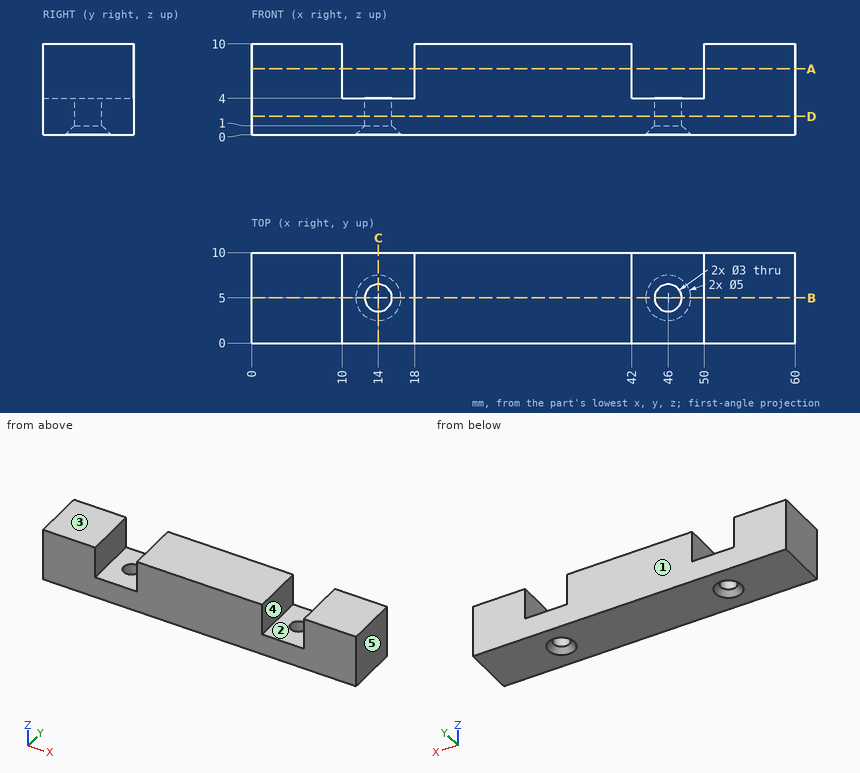
Here's the drawing with two shaded views (mm, measured from the low corner). I have some questions. A direction names the side the tool comes from. Coordinates: 2 decimals unless noted, no trailing zeros. Order: outer loops, then holes, each group sorted by start corner. A loop starts at its lowest first (then second) coordinate and runs counter-clockwise, first axis right, second up.
Item 1: For the marked faces 1 and 2, which set-ups out of +Z, -Z, +X, -X, +Y, -Y let a thin tool reach every point of the face, with its end or its side?
Result sheet:
face 1: +Z, -Z, +X, -X, +Y
face 2: +Z, +Y, -Y
Item 2: For P1, Ø4, axis at x = 13.5, y = 4.5, coming from the +Z side; P2, Ø3, axis at y = 7.5, z = 8, coming from the -X side, each with a flat end and sliding along its axis, tell me the tip position at first contact or that it passes through.
Result sheet:
P1: stops at z = 4
P2: stops at x = 0
Item 3: If we section it at D-D on z = 2: List the corners of the cut face in (x, y) for me.
Result sheet:
outline: (0, 0) - (60, 0) - (60, 10) - (0, 10) - close; hole circle Ø3 at (14, 5); hole circle Ø3 at (46, 5)
Item 4: If we section it at C-C on x = 14: List the corners of the cut face in (y, z) for me, plus the area to 3 significant figures.
Result sheet:
outline: (0, 0) - (2.5, 0) - (3.5, 1) - (3.5, 4) - (0, 4) - close; (6.5, 1) - (7.5, 0) - (10, 0) - (10, 4) - (6.5, 4) - close
area: 27.0 mm2
Item 5: If we section it at B-B on y = 5: List the corners of the cut face in (x, z) for me, plus the area to 3 significant figures.
Result sheet:
outline: (0, 0) - (11.5, 0) - (12.5, 1) - (12.5, 4) - (10, 4) - (10, 10) - (0, 10) - close; (15.5, 1) - (16.5, 0) - (43.5, 0) - (44.5, 1) - (44.5, 4) - (42, 4) - (42, 10) - (18, 10) - (18, 4) - (15.5, 4) - close; (47.5, 1) - (48.5, 0) - (60, 0) - (60, 10) - (50, 10) - (50, 4) - (47.5, 4) - close
area: 478 mm2
Item 6: If we section it at A-A on z = 7.25: List the corners of the cut face in (x, y) for me, plus the area to 3 significant figures.
Result sheet:
outline: (0, 0) - (10, 0) - (10, 10) - (0, 10) - close; (18, 0) - (42, 0) - (42, 10) - (18, 10) - close; (50, 0) - (60, 0) - (60, 10) - (50, 10) - close
area: 440 mm2
Item 7: I need wall thicknesses on line 1 (X direction, y = 3, z = 8); line 2 (X direction, y = 5, z = 2.15); line 3 (Y direction, x = 14, z = 3.15). Which ranges of each line are inside material? Lowest first, please.
Result sheet:
line 1: x = 0 to 10, 18 to 42, 50 to 60
line 2: x = 0 to 12.5, 15.5 to 44.5, 47.5 to 60
line 3: y = 0 to 3.5, 6.5 to 10
Item 8: If we mould it in two halves opening along X, with no side actions, what happens to the marked faces 3, 4 and 5? For each: +X half, -X half, draft (parallel to the pull), parting line (faces both ways), or undercut.
Result sheet:
face 3: draft
face 4: undercut
face 5: +X half
